Geometry check sheet. Reference: the model listing, model coordinates, mm. A direction names the side the tool comes from. Round coordinates to 2 decimals unless told otherwise and drop trailing zeros. Write each loop counter-clockwise with the first axis right and the second up, starting at its lowest first coordinate (ties: lowest second). Pieces come first, ordered by that corner, then holes.
Item 1: Depth check by flat-ended pin: P1, Ø3, axis at x = 0, y = -11.58, coming from the +Z side (3 decimals); P2, Ø2, axis at x = -18, y = 5.5, coming from the +Z side. Enter the tip coordinate at first touch or a pass-through.
Item 2: Cross-section at A-A (y = 0). Enter the section's corners in (x, z) (3 decimals).
Item 3: Cross-section at D-D (z = 3.5). State how many separate pieces and enclosed holes the cut face has, then the cut area to 3 significant figures.
Item 4: Cross-section at C-C (x = 33). Enter the section's corners in (y, z), then the cut area to 3 significant figures.
Item 5: Cross-section at B-B (x = 0). Enter the section's corners in (y, z), then the cut area to 3 significant figures.
Item 6: Access from +Z, -Z, +X, -X, +Y, -Y to the whole of each face (thin tool, end or side, straight path). Record for faces 1 (the face through (-17.47, -1.22, 2.46)), 2 (the face through (-16, -9, 7)).
Item 7: Scan lines: probe 1 along Y at (x, z) = (33, 7.25); probe 2 along X at (y, z) = (-4, 9); probe 3 along Y at (x, z) = (-23, 6). Record each from-to range of solid material in increasing order.
from build123d import *

# Parameters (mm, degrees)
F0_W     = 71
F0_H     = 28
F0_R     = 1.55
F0_W_2   = 2
F0_H_2   = 1
F1_DEPTH = 9.65
F0_R_2   = 3.25
F0_R_3   = 3.175
F2_DEPTH = 5
F3_R     = 0.99999


# Not quite as in the source:
# - a fillet or chamfer is up to 0.001 mm smaller than in the source, because OpenCascade refuses the exact size


with BuildPart() as f1:
    # F0 (on Top) → F1 (new body)
    with BuildSketch(Plane.XY):
        Rectangle(F0_W, F0_H)
        with Locations((-33, -11.5)):
            Circle(F0_R, mode=Mode.SUBTRACT)
        with Locations((-16.5, -11.5939453244)):
            Circle(F0_R, mode=Mode.SUBTRACT)
        with Locations((0, -11.5801189095)):
            Circle(F0_R, mode=Mode.SUBTRACT)
        with Locations((16.5, -11.5939453244)):
            Circle(F0_R, mode=Mode.SUBTRACT)
        with Locations((33, -11.5)):
            Circle(F0_R, mode=Mode.SUBTRACT)
        with Locations((-33, 11.5)):
            Circle(F0_R, mode=Mode.SUBTRACT)
        with Locations((-16.5, 11.5939453244)):
            Circle(F0_R, mode=Mode.SUBTRACT)
        Polygon((-30.5, -9), (-30.5, 9), (-1, 9), (1, 9), (30.5, 9), (30.5, -9), (1, -9), (-1, -9), align=None, mode=Mode.SUBTRACT)
        with Locations((0, 11.5801189095)):
            Circle(F0_R, mode=Mode.SUBTRACT)
        with Locations((16.5, 11.5939453244)):
            Circle(F0_R, mode=Mode.SUBTRACT)
        with Locations((33, 11.5)):
            Circle(F0_R, mode=Mode.SUBTRACT)
        with Locations((0, -8.5)):
            Rectangle(F0_W_2, F0_H_2)
        with Locations((0, 8.5)):
            Rectangle(F0_W_2, F0_H_2)
    extrude(amount=F1_DEPTH)

    # F0 (on Top) → F2 (join)
    with BuildSketch(Plane.XY):
        Polygon((30.5, 9), (1, 9), (1, 8), (1, 0), (1, -8), (1, -9), (30.5, -9), align=None)
        with Locations((9, 0)):
            Circle(F0_R_2, mode=Mode.SUBTRACT)
        with Locations((20.4, 0)):
            Circle(F0_R_3, mode=Mode.SUBTRACT)
        Polygon((-1, 9), (-30.5, 9), (-30.5, -9), (-1, -9), (-1, -8), (-1, -6.4e-09), (-1, 8), align=None)
        with Locations((-20.4, 0)):
            Circle(F0_R_3, mode=Mode.SUBTRACT)
        with Locations((-9, 0)):
            Circle(F0_R_3, mode=Mode.SUBTRACT)
        with BuildLine():
            ThreePointArc((1, 0), (3.2e-09, -1), (-1, -6.4e-09))
            Line((-1, -6.4e-09), (-1, -8))
            Line((-1, -8), (1, -8))
            Line((1, -8), (1, 0))
        make_face()
        with BuildLine():
            Line((1, 8), (-1, 8))
            Line((-1, 8), (-1, -6.4e-09))
            ThreePointArc((-1, -6.4e-09), (-3.2e-09, 1), (1, 0))
            Line((1, 0), (1, 8))
        make_face()
    extrude(amount=F2_DEPTH)

    # F3 (radius 1 in the source; OpenCascade refuses exactly that, so slightly less here)
    f3_edges = [f1.edges().sort_by_distance(p)[0] for p in [
        (-30.5, -9, 7.325),
        (-1, -9, 7.325),
        (-30.5, 9, 7.325),
        (-1, 9, 7.325),
        (1, 9, 7.325),
        (1, -9, 7.325),
        (30.5, -9, 7.325),
        (30.5, 9, 7.325),
    ]]
    fillet(f3_edges, radius=F3_R)


solid = f1.part
Resolved:
1. P1: passes through
1. P2: stops at z = 5
2. outline: (-35.5, 0) - (-23.575, 0) - (-23.575, 5) - (-30.5, 5) - (-30.5, 9.65) - (-35.5, 9.65) - close; (-17.225, 0) - (-12.175, 0) - (-12.175, 5) - (-17.225, 5) - close; (-5.825, 0) - (-1, 0) - (-1, 5) - (-5.825, 5) - close; (1, 0) - (5.75, 0) - (5.75, 5) - (1, 5) - close; (12.25, 0) - (17.225, 0) - (17.225, 5) - (12.25, 5) - close; (23.575, 0) - (35.5, 0) - (35.5, 9.65) - (30.5, 9.65) - (30.5, 5) - (23.575, 5) - close
3. separate pieces: 1
3. enclosed holes: 15
3. area: 1,780 mm2
4. outline: (-14, 0) - (-13.05, 0) - (-13.05, 9.65) - (-14, 9.65) - close; (-9.95, 0) - (9.95, 0) - (9.95, 9.65) - (-9.95, 9.65) - close; (13.05, 0) - (14, 0) - (14, 9.65) - (13.05, 9.65) - close
4. area: 210 mm2
5. outline: (-14, 0) - (-13.13, 0) - (-13.13, 9.65) - (-14, 9.65) - close; (-10.03, 0) - (-1, 0) - (-1, 5) - (-8, 5) - (-8, 9.65) - (-10.03, 9.65) - close; (1, 0) - (10.03, 0) - (10.03, 9.65) - (8, 9.65) - (8, 5) - (1, 5) - close; (13.13, 0) - (14, 0) - (14, 9.65) - (13.13, 9.65) - close
5. area: 126 mm2
6. face 1: +Z, -Z
6. face 2: +Z
7. probe 1: y = -14 to -13.05, -9.95 to 9.95, 13.05 to 14
7. probe 2: x = -35.5 to -30.5, 30.5 to 35.5
7. probe 3: y = -14 to -9, 9 to 14
